Geometry: final body of the model. Coordinates: model frame, mm. Face numbers are marked on the shaded views. A direction names the side the tool comes from. Give positions to 0.01 mm unless a question says otherwise; leave off trailing zeros. Order: outer loops, then holes, each group sorted by start corner. A loop starts at its lowest first (then second) coordinate and runs counter-clockwise, first axis right, second up. Notation, with made-up numbers: (75.25, -7.75) -> (85.25, -7.75) arc R7 cw to (85.25, 1.25) -> close; hole circle Ø3 at (-8, 27). An arc over 180 degrees is marked (long way). Answer in a Markdown table with one row per item. Add a question column.
Q1. Cut plane C-C on z = -6.5. Return the cut outline in (x, y), and give its area (3 significant figures).
Q2. Cut plane B-B on z = 0. Return the cut outline in (x, y), and give its area (3 significant figures).
Q3. Cut plane A-A on x = -25.4. Return the cut outline in (y, z), and give its area (3 significant figures).
Q4. Contact query for flat-ended pins moving along their axis: P1, Ø6, axis at x = 15, z = 8.5, coming from the -Y side; P2, Ø3.5, axis at x = 25.4, z = 0, coming from the -Y side. Output: stop coordinate, or through.
Q5. Set-up query: the marked faces 1, 2 and 3. Return all of +Z, -Z, +X, -X, +Y, -Y with unobstructed straight access to the full face (end or side cutting, diameter ignored); none if empty.
Q6. Pull-direction query (Z, two-part tool) for the marked faces 4, 5 and 6; classes: +Z half, -Z half, draft (parallel to the pull), parting line (faces both ways), or undercut.
Q7. Line query: line 1 along Z through (x, y) = (1, 4.75); line 2 along Z through (x, y) = (25.4, 5.05); line 3 along Y through (x, z) = (-27, 9.5). Output: solid intervals per line, ascending. Write a range as from..to.
Q8. Cut plane D-D on y = 1. Return the cut outline in (x, z).
from build123d import *

# Parameters (mm, degrees)
SKETCH1_W               = 76.2
SKETCH1_H               = 26.162
BOSS_EXTRUDE1_DEPTH     = 6.35
FILLET1_R               = 4.826
SKETCH2_W               = 22.225
SKETCH2_H               = 1.651
CUT_EXTRUDE1_DEPTH      = 78.574964138
CUT_EXTRUDE2_DEPTH      = 41.556172921
CUT_EXTRUDE2_DEPTH_BACK = 41.556172921
F_4_40_TAPPED_HOLE1_D   = 2.2606


with BuildPart() as part:
    # Sketch1 → Boss-Extrude1 (new body)
    with BuildSketch(Plane(origin=(0, 0, 0), x_dir=(1, 0, 0), z_dir=(0, 1, 0))):
        Rectangle(SKETCH1_W, SKETCH1_H)
    extrude(amount=BOSS_EXTRUDE1_DEPTH)

    # Fillet1
    fillet1_edges = [part.edges().sort_by_distance(p)[0] for p in [
        (-38.1, 0, 0),
        (38.1, 0, 0),
    ]]
    fillet(fillet1_edges, radius=FILLET1_R)

    # Sketch2 → Cut-Extrude1 (cut, through all)
    with BuildSketch(Plane(origin=(38.1, 0, 0), x_dir=(0, 0, -1), z_dir=(1, 0, 0))):
        with Locations((0, 0.8255)):
            Rectangle(SKETCH2_W, SKETCH2_H)
    extrude(amount=-CUT_EXTRUDE1_DEPTH, mode=Mode.SUBTRACT)

    # Sketch3 → Cut-Extrude2 (cut, two sides: drawn at the far end of the back side and taken through both)
    with BuildSketch(Plane.XZ.offset(-1.651).offset(-CUT_EXTRUDE2_DEPTH_BACK)):
        with BuildLine():
            Line((6.7945, -11.1125), (-6.7945, -11.1125))
            ThreePointArc((-6.7945, -11.1125), (-8.051735857, -10.591735857), (-8.5725, -9.3345))
            Line((-8.5725, -9.3345), (-8.5725, 9.3345))
            ThreePointArc((-8.5725, 9.3345), (-8.051735857, 10.591735857), (-6.7945, 11.1125))
            Line((-6.7945, 11.1125), (6.7945, 11.1125))
            ThreePointArc((6.7945, 11.1125), (8.051735857, 10.591735857), (8.5725, 9.3345))
            Line((8.5725, 9.3345), (8.5725, -9.3345))
            ThreePointArc((8.5725, -9.3345), (8.051735857, -10.591735857), (6.7945, -11.1125))
        make_face()
    extrude(amount=CUT_EXTRUDE2_DEPTH + CUT_EXTRUDE2_DEPTH_BACK, mode=Mode.SUBTRACT)

    # #4-40 Tapped Hole1 (through all)
    with Locations(Plane(origin=(0, 6.35, 0), x_dir=(-1, 0, 0), z_dir=(0, 1, 0))):
        with Locations((25.4, 0), (-25.4, 0)):
            Hole(F_4_40_TAPPED_HOLE1_D / 2)


solid = part.part
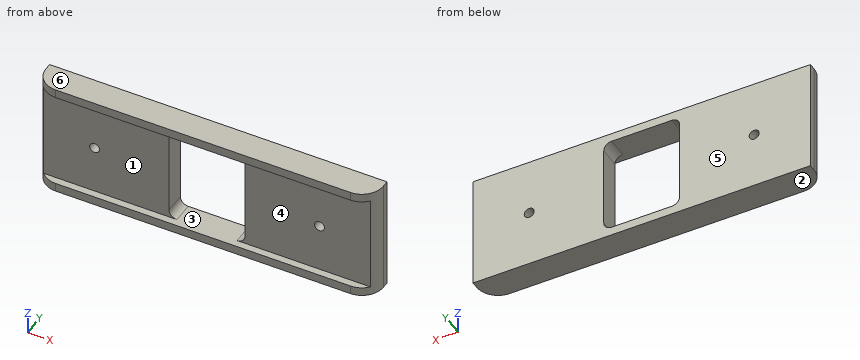
Completed:
| question | item | result |
|---|---|---|
| 1 | outline | (-38.1, 4.83) arc R4.83 ccw to (-36.91, 1.65) -> (-8.57, 1.65) -> (-8.57, 6.35) -> (-38.1, 6.35) -> close; (8.57, 1.65) -> (36.91, 1.65) arc R4.83 ccw to (38.1, 4.83) -> (38.1, 6.35) -> (8.57, 6.35) -> close |
| 1 | area | 275 mm² |
| 2 | outline | (-38.1, 4.83) arc R4.83 ccw to (-36.91, 1.65) -> (-26.53, 1.65) -> (-26.53, 6.35) -> (-38.1, 6.35) -> close; (-24.27, 1.65) -> (-8.57, 1.65) -> (-8.57, 6.35) -> (-24.27, 6.35) -> close; (8.57, 1.65) -> (24.27, 1.65) -> (24.27, 6.35) -> (8.57, 6.35) -> close; (26.53, 1.65) -> (36.91, 1.65) arc R4.83 ccw to (38.1, 4.83) -> (38.1, 6.35) -> (26.53, 6.35) -> close |
| 2 | area | 254 mm² |
| 3 | outline | (0, -13.08) -> (6.35, -13.08) -> (6.35, -1.13) -> (1.65, -1.13) -> (1.65, -11.11) -> (0, -11.11) -> close; (0, 11.11) -> (1.65, 11.11) -> (1.65, 1.13) -> (6.35, 1.13) -> (6.35, 13.08) -> (0, 13.08) -> close |
| 3 | area | 119 mm² |
| 4 | P1 | stops at y = 0 |
| 4 | P2 | stops at y = 1.65 |
| 5 | face 1 | +X, -X, -Y |
| 5 | face 2 | -Z, +X, -X, +Y, -Y |
| 5 | face 3 | -Y |
| 6 | face 4 | undercut |
| 6 | face 5 | draft |
| 6 | face 6 | +Z half |
| 7 | line 1 | z = -13.08..-11.11, 11.11..13.08 |
| 7 | line 2 | z = -13.08..-1.13, 1.13..13.08 |
| 7 | line 3 | y = 1.65..6.35 |
| 8 | outline | (-36.22, -13.08) -> (36.22, -13.08) -> (36.22, -11.11) -> (-36.22, -11.11) -> close; (-36.22, 11.11) -> (36.22, 11.11) -> (36.22, 13.08) -> (-36.22, 13.08) -> close |
